from build123d import *

# Parameters (mm, degrees)
F1_DEPTH = 63.5
F2_DEPTH = 12.7
F0_W     = 25.4
F0_H     = 19.05
F3_DEPTH = 25.4


with BuildPart() as f1:
    # F0 (on Front) → F1 (new body, symmetric)
    with BuildSketch(Plane.XZ):
        Polygon((38.1, -12.7), (38.1, 12.7), (19.05, 12.7), (-38.1, 12.7), (-38.1, -12.7), align=None)
    extrude(amount=F1_DEPTH, both=True)

    # F0 (on Front) → F2 (join, symmetric)
    with BuildSketch(Plane.XZ):
        with BuildLine():
            Line((-38.1, 12.7), (19.05, 12.7))
            Line((19.05, 12.7), (19.05, 24.765))
            ThreePointArc((19.05, 24.765), (28.9881633288, 49.1660987082), (53.1466996803, 59.6801764077))
            add(Edge.make_bspline(
                [(-38.1, 12.7), (-38.4659506113, 42.7773494119), (-9.3436090352, 58.8699288364), (53.1466996803, 59.6801764077)],
                knots=[0, 0, 0, 0, 102.9188043099, 102.9188043099, 102.9188043099, 102.9188043099], degree=3))
        make_face()
    extrude(amount=F2_DEPTH, both=True)

    # F0 (on Front) → F3 (join, symmetric)
    with BuildSketch(Plane.XZ):
        with BuildLine():
            Line((19.05, 12.7), (38.1, 12.7))
            Line((38.1, 12.7), (38.1, 24.765))
            ThreePointArc((38.1, 24.765), (42.7496798487, 35.9903201513), (53.975, 40.64))
            Line((53.975, 40.64), (63.5, 40.64))
            Line((63.5, 40.64), (63.5, 59.69))
            Line((63.5, 59.69), (53.975, 59.69))
            add(Edge.make_bspline(
                [(53.1466996803, 59.6801764077), (53.4221513474, 59.6837479062), (53.6982513432, 59.687022474), (53.975, 59.69)],
                knots=[102.9188043099, 102.9188043099, 102.9188043099, 102.9188043099, 103.3724611538, 103.3724611538, 103.3724611538, 103.3724611538], degree=3))
            ThreePointArc((53.1466996803, 59.6801764077), (28.9881633288, 49.1660987082), (19.05, 24.765))
            Line((19.05, 24.765), (19.05, 12.7))
        make_face()
        with Locations((76.2, 50.165)):
            Rectangle(F0_W, F0_H)
    extrude(amount=F3_DEPTH, both=True)

    # F0 (on Front) → F4 (revolve)
    with BuildSketch(Plane.XZ):
        Polygon((88.9, 59.69), (88.9, 40.64), (88.9, 38.1), (114.3, 38.1), (114.3, 63.5), (88.9, 63.5), align=None)
    revolve(axis=Axis((88.9, 0, 50.8), (0, 0, -1)))


solid = f1.part
The model under review builds one solid part; all positions refer to its coordinate system, in mm. A direction names the side the tool comes from. Coordinates: 2 decimals unless noted, no trailing zeros. Loops run counter-clockwise (first coordinate to the right, second up) from the corner with the lowest first, then second, coordinate; pieces in that order, holes last. Notation, with made-up numbers: M 50.5,-13.5 L 98.5,-13.5 A31 cw 98.5,12.5 Z; hole C 72,9 d7. An arc over 180 degrees is marked long. Put each result on its own line as item: value. Start each with the question number.
Q1. For faces 4 (the cylindrical face through (29.254, -19.139, 49.435)), 5 (the cylindrical face through (29.254, 18.961, 49.435)), 6 (the flat face through (60, 0, 59.69)), 7 (the flat face through (38.1, -1, 2)), list the 3-axis set-ups (+Z, -Z, +X, -X, +Y, -Y) from which the entire face can be reached by the end or side of a thin tool; tool diameter is ignored.
Q2. The part is to be moulded in two halves that separate along X. For faces 1 (the flat face through (-3, -12.7, 31)), 2 (the flat face through (19.05, 19, 19)), 3 (the flat face through (63, 0, 40.64)), say which applies: +X half, -X half, draft (parallel to the pull), parting line (faces both ways), or undercut.
Q3. Clearance check with flat-ended pins moving along their axes: pin 1 (12 mm diameter, centred on y = 43.5, z = -4.5, fed in from -X); pin 2 (9.5 mm diameter, centred on y = 20.5, z = 20.5, fed in from -X); pin 3 (8 mm diameter, centred on y = -48, z = 14, fed in from +X). State where each tip first meets the part, or that it passes through.
Q4. Add section A-A (z = -0.5). Write out the cut boundary in (x, y).
Q5. Wall thickness on line 1 (X direction, y = -16.5, z = 2); line 2 (Z direction, x = 87, y = -11); line 3 (Y direction, x = 8, z = 38): over which ranges is each line inside the solid? List them lowest first.
Q6. Add section B-B (y = 35). Write out the cut boundary in (x, z).
Answers:
1. face 4: +Z, -X, -Y
1. face 5: +Z, -X, +Y
1. face 6: +Z, -X
1. face 7: -Z, +X, +Y, -Y
2. face 1: draft
2. face 2: -X half
2. face 3: undercut
3. pin 1: stops at x = -38.1
3. pin 2: stops at x = 19.05
3. pin 3: stops at x = 38.1
4. outline: M -38.1,-63.5 L 38.1,-63.5 L 38.1,63.5 L -38.1,63.5 Z
5. line 1: x = -38.1 to 38.1
5. line 2: z = 38.1 to 63.5
5. line 3: y = -12.7 to 12.7
6. outline: M -38.1,-12.7 L 38.1,-12.7 L 38.1,12.7 L -38.1,12.7 Z
